CAD build for the part. Positions are in the model's coordinates, mm. A direction names the side the tool comes from. Give positions to 0.01 mm unless a question says otherwise; leave off trailing zeros. Loops run counter-clockwise (first coordinate to the right, second up) from the corner with the lowest first, then second, coordinate; pieces in that order, holes last. Notation, with made-up numbers: M -6.5,83.25 L -1.5,83.25 A34 ccw -1.5,122.25 Z; hole C 45,5 d11. An arc over 180 degrees is marked long. One line per question, with ' | ' between items.
```python
from build123d import *

# Parameters (mm, degrees)
BOSS_EXTRUDE1_DEPTH = 2.5
SKETCH2_W           = 15
SKETCH2_H           = 2.5
BOSS_EXTRUDE2_DEPTH = 3
SKETCH5_R           = 1.524
BOSS_EXTRUDE4_DEPTH = 2.5
SKETCH6_R           = 1.524
CUT_EXTRUDE1_DEPTH  = 2.5
SKETCH7_R           = 1.5
CUT_EXTRUDE2_DEPTH  = 2.5


with BuildPart() as part:
    # Sketch1 → Boss-Extrude1 (new body)
    with BuildSketch(Plane(origin=(0, 0, 0), x_dir=(1, 0, 0), z_dir=(0, 1, 0))):
        Polygon((-87, -50), (-87, -7.25), (-112, -7.25), (-112, 7.25), (-87, 7.25), (-87, 50), (87, 50), (87, -50), align=None)
    extrude(amount=BOSS_EXTRUDE1_DEPTH)

    # Sketch2 → Boss-Extrude2 (add)
    with BuildSketch(Plane.XY.offset(50)):
        with Locations((-63.5, 1.25)):
            Rectangle(SKETCH2_W, SKETCH2_H)
        with Locations((63.5, 1.25)):
            Rectangle(SKETCH2_W, SKETCH2_H)
    boss_extrude2 = extrude(amount=BOSS_EXTRUDE2_DEPTH)

    # Mirror1: Boss-Extrude2 across plane
    add(boss_extrude2.mirror(Plane.XY))

    # Sketch5 → Boss-Extrude4 (add)
    with BuildSketch(Plane(origin=(0, 2.5, 0), x_dir=(1, 0, 0), z_dir=(0, 1, 0))):
        with BuildLine():
            Line((-102.204774668, -46.50231683), (-94.729060006, -33.553999212))
            Line((-94.729060006, -33.553999212), (-87, -33.553999212))
            Line((-87, -33.553999212), (-87, -18.493123836))
            Line((-87, -18.493123836), (-102.458120011, -18.493123836))
            Line((-102.458120011, -18.493123836), (-114.523120011, -39.39031683))
            ThreePointArc((-114.523120011, -39.39031683), (-111.919947339, -49.105489501), (-102.204774668, -46.50231683))
        make_face()
        with Locations(Location((-99.854947339, -28.208296508, 0), (0, 0, 270))):
            Circle(SKETCH5_R, mode=Mode.SUBTRACT)
    boss_extrude4 = extrude(amount=-BOSS_EXTRUDE4_DEPTH)

    # Sketch6 → Cut-Extrude1 (cut)
    with BuildSketch(Plane.XZ):
        with Locations(Location((-87.318751132, 0, 0), (0, 0, 270))):
            Circle(SKETCH6_R)
    extrude(amount=-CUT_EXTRUDE1_DEPTH, mode=Mode.SUBTRACT)

    # Mirror2: Boss-Extrude4 across plane
    add(boss_extrude4.mirror(Plane.XY))

    # Sketch7 → Cut-Extrude2 (cut)
    with BuildSketch(Plane(origin=(0, 2.5, 0), x_dir=(1, 0, 0), z_dir=(0, 1, 0))):
        with BuildLine():
            ThreePointArc((-57, -43), (-55.5, -44.5), (-57, -46))
            Line((-57, -46), (-72, -46))
            ThreePointArc((-72, -46), (-73.5, -44.5), (-72, -43))
            Line((-72, -43), (-57, -43))
        make_face()
        with BuildLine():
            Line((-17.5, -46), (-7.5, -46))
            ThreePointArc((-7.5, -46), (-6, -44.5), (-7.5, -43))
            Line((-7.5, -43), (-17.5, -43))
            ThreePointArc((-17.5, -43), (-19, -44.5), (-17.5, -46))
        make_face()
        with BuildLine():
            Line((-72, 43), (-57, 43))
            ThreePointArc((-57, 43), (-55.5, 44.5), (-57, 46))
            Line((-57, 46), (-72, 46))
            ThreePointArc((-72, 46), (-73.5, 44.5), (-72, 43))
        make_face()
        with BuildLine():
            ThreePointArc((-7.5, 46), (-6, 44.5), (-7.5, 43))
            Line((-7.5, 43), (-17.5, 43))
            ThreePointArc((-17.5, 43), (-19, 44.5), (-17.5, 46))
            Line((-17.5, 46), (-7.5, 46))
        make_face()
        with Locations(Location((0, 44.5, 0), (0, 0, 270))):
            Circle(SKETCH7_R)
        with Locations(Location((0, -44.5, 0), (0, 0, 270))):
            Circle(SKETCH7_R)
    extrude(amount=-CUT_EXTRUDE2_DEPTH, mode=Mode.SUBTRACT)


solid = part.part
```
Item 1: Mould opens along X. For faces 1 (the flat face through (-98.52, 1.27, 40.12)), 2 (the flat face through (-108.41, 1.27, -28.8)), 3 (the flat face through (-13, 0, -1)) say: pulls with the +X half, pulls with the -X half, needs draft (parallel to the pull), parting line crosses it, or undercut.
Conclusion:
face 1: undercut | face 2: pulls with the -X half | face 3: needs draft
Item 2: Drop flat-ended pins along their axis: P1, Ø0.8, axis at x = -11, y = 1, coming from the +Z side; P2, Ø1.2, axis at x = -91, y = 2, coming from the +Z side; P3, Ø1.5, axis at y = 0.5, z = -35.5, coming from the -X side. Give the stop position or say it passes through.
Conclusion:
P1: z = 50 | P2: z = 33.55 | P3: x = -112.71
Item 3: Saw through at A-A on x = -27. Give the cut face in (y, z), and give its area (3 significant figures).
Conclusion:
outline: M 0,-50 L 2.5,-50 L 2.5,50 L 0,50 Z | area: 250 mm²
Item 4: Saw through at C-C on y = 0.8. State how many separate pieces and enclosed holes the cut face has, and give its area (3 significant figures).
Conclusion:
separate pieces: 1 | enclosed holes: 9 | area: 18,800 mm²
Item 5: Drill centre lines: line 1 along Z through (x, y) = (-15, 2.25); line 2 along Z through (x, y) = (-62, 0.5); line 3 along X through (y, z) = (1.55, 44.5). Where is each one in solid material? Low to high. Write a range as [from, to].
Conclusion:
line 1: [-50, -46], [-43, 43], [46, 50] | line 2: [-53, -46], [-43, 43], [46, 53] | line 3: [-115.3, -101.05], [-87, -73.5], [-55.5, -19], [-6, -1.5], [1.5, 87]
Item 6: Saw through at B-B on z = 22. Give the cut face in (x, y).
Conclusion:
outline: M -104.48,0 L 87,0 L 87,2.5 L -104.48,2.5 Z
Item 7: 3-axis set-ups, long thin cutter, end or side, ignore diameter. For faces 4 (the flat face through (-108.41, 1.27, 28.8)), 5 (the cylindrical face through (-112.1, 1.3, 49)), 6 (the flat face through (-98.52, 1.27, -40.12)): which of +Z, -Z, +X, -X, +Y, -Y reach the whole face in a straight line?
Conclusion:
face 4: -X, +Y, -Y | face 5: +Y, -Y | face 6: -Z, +Y, -Y
